Geometry: final body of the model. Coordinates: model frame, mm. A direction names the side the tool comes from. Coordinates: 2 decimals unless noted, no trailing zeros. Loops run counter-clockwise (first coordinate to the right, second up) from the corner with the lowest first, then second, coordinate; pieces in that order, holes last. Notation, with made-up numbers: (57.25, 10.5) - (79.25, 10.5) arc R21 ccw to (79.25, 46.5) - close; hole circle Ø6 at (26, -19). An arc over 180 degrees is marked (long way). Put each result on its own line as item: value. Start each with the question number.
1) Reachability of faces 3 (the cylindrical face through (-25, 16, 2)), 4 (the flat face through (-2, 1, 5)), 5 (the flat face through (-124, -41, 2)), 6 (the flat face through (95, 0, 2)), 7 (the flat face through (-120, -66, 2)) from +Z, -Z, +X, -X, +Y, -Y: full face, straight path, thin tool, end or side. Return the list, or none.
2) Material intervals for line 1 along X through (y, z) = (2.5, 4.7); line 2 along X through (y, z) = (-15, 4.5); line 3 along X through (y, z) = (-39, 0.7), sorted ascending. Write a range as from..to.
3) Section C-C on y = -20.5. Output: boundary loops of the cut face in (x, z), and give its area (3 significant figures).
4) Draft query along Y for faces 1 (the flat face through (120, 65, 2)), 2 (the flat face through (103, -2.2, 2)). Return one class per face: +Y half, -Y half, draft (parallel to the pull), parting line (faces both ways), or undercut.
5) Contact query for flat-ended pins moving along their axis: pin 1 Ø3 at (x, y) = (-37.5, -70.5) entering from +Z; pin 2 Ø5.5 at (x, y) = (-92, 23.5) entering from -Z; pin 3 Ø0.8 at (y, z) = (-3, 1.5) entering from -X; pin 4 Ø2.5 at (y, z) = (-2.5, 3) entering from +X. Output: stop coordinate, or through.
6) Section B-B on x = -12. Output: boundary loops of the cut face in (y, z), and give its area (3 significant figures).
7) Section A-A on y = 12. Output: boundary loops of the cut face in (x, z), and give its area (3 significant figures).
8) Section D-D on x = 91. Output: boundary loops of the cut face in (y, z), and give its area (3 significant figures).
```python
from build123d import *

# Parameters (mm, degrees)
SKETCH1_W           = 240
SKETCH1_H           = 151
BOSS_EXTRUDE1_DEPTH = 5
SKETCH2_R           = 1.25
CUT_EXTRUDE1_DEPTH  = 5
CUT_EXTRUDE2_DEPTH  = 10
SKETCH7_R           = 2
CUT_EXTRUDE4_DEPTH  = 10
SKETCH9_W           = 4
SKETCH9_H           = 30
BOSS_EXTRUDE2_DEPTH = 5
CUT_EXTRUDE6_DEPTH  = 5
SKETCH13_R          = 21
CUT_EXTRUDE9_DEPTH  = 10
SKETCH15_R          = 1.75
CUT_EXTRUDE11_DEPTH = 10
SKETCH16_R          = 1.75
CUT_EXTRUDE12_DEPTH = 10
SKETCH17_R          = 1.75
CUT_EXTRUDE13_DEPTH = 10
SKETCH20_W          = 24.2
SKETCH20_H          = 30.2
CUT_EXTRUDE14_DEPTH = 10
SKETCH21_R          = 5.25
CUT_EXTRUDE15_DEPTH = 5
SKETCH22_R          = 1
CUT_EXTRUDE16_DEPTH = 5
SKETCH23_R          = 5.25
CUT_EXTRUDE17_DEPTH = 10


with BuildPart() as part:
    # Sketch1 → Boss-Extrude1 (new body)
    with BuildSketch(Plane.XY):
        Rectangle(SKETCH1_W, SKETCH1_H)
    extrude(amount=BOSS_EXTRUDE1_DEPTH)

    # Sketch2 → Cut-Extrude1 (cut)
    with BuildSketch(Plane(origin=(0, 0, 0), x_dir=(-1, 0, 0), z_dir=(0, 0, -1))):
        with Locations(Location((-20, 42, 0), (0, 0, 180))):
            Circle(SKETCH2_R)
        with Locations((28, 28)):
            Circle(SKETCH2_R)
        with Locations(Location((20, 42, 0), (0, 0, 180))):
            Circle(SKETCH2_R)
        with Locations((-28, 28)):
            Circle(SKETCH2_R)
        with Locations(Location((-28, -28, 0), (0, 0, 180))):
            Circle(SKETCH2_R)
        with Locations((20, -42)):
            Circle(SKETCH2_R)
        with Locations(Location((28, -28, 0), (0, 0, 180))):
            Circle(SKETCH2_R)
        with Locations((-20, -42)):
            Circle(SKETCH2_R)
    extrude(amount=-CUT_EXTRUDE1_DEPTH, mode=Mode.SUBTRACT)

    # Sketch5 → Cut-Extrude2 (cut)
    with BuildSketch(Plane(origin=(0, 0, 0), x_dir=(-1, 0, 0), z_dir=(0, 0, -1))):
        with BuildLine():
            Line((18.5, -10.5), (18.5, 9.5))
            ThreePointArc((18.5, 9.5), (25, 16), (31.5, 9.5))
            Line((31.5, 9.5), (31.5, -10.5))
            ThreePointArc((31.5, -10.5), (25, -17), (18.5, -10.5))
        make_face()
        with BuildLine():
            Line((-18.5, -10.5), (-18.5, 9.5))
            ThreePointArc((-18.5, 9.5), (-25, 16), (-31.5, 9.5))
            Line((-31.5, 9.5), (-31.5, -10.5))
            ThreePointArc((-31.5, -10.5), (-25, -17), (-18.5, -10.5))
        make_face()
    extrude(amount=-CUT_EXTRUDE2_DEPTH, mode=Mode.SUBTRACT)

    # Sketch7 → Cut-Extrude4 (cut)
    with BuildSketch(Plane(origin=(0, 0, 0), x_dir=(-1, 0, 0), z_dir=(0, 0, -1))):
        with Locations((29.207613065, 40.217347852)):
            Circle(SKETCH7_R)
        with Locations((29.207613065, -40.217347852)):
            Circle(SKETCH7_R)
        with Locations(Location((-29.207613065, -40.217347852, 0), (0, 0, 180))):
            Circle(SKETCH7_R)
        with Locations(Location((-29.207613065, 40.217347852, 0), (0, 0, 180))):
            Circle(SKETCH7_R)
    extrude(amount=-CUT_EXTRUDE4_DEPTH, mode=Mode.SUBTRACT)

    # Sketch9 → Boss-Extrude2 (add)
    with BuildSketch(Plane(origin=(0, 0, 0), x_dir=(-1, 0, 0), z_dir=(0, 0, -1))):
        with Locations((122, 40.5)):
            Rectangle(SKETCH9_W, SKETCH9_H)
        with Locations((122, -40.5)):
            Rectangle(SKETCH9_W, SKETCH9_H)
        with Locations((-122, -40.5)):
            Rectangle(SKETCH9_W, SKETCH9_H)
        with Locations((-122, 40.5)):
            Rectangle(SKETCH9_W, SKETCH9_H)
    extrude(amount=-BOSS_EXTRUDE2_DEPTH)

    # Sketch10 → Cut-Extrude6 (cut)
    with BuildSketch(Plane(origin=(0, 0, 0), x_dir=(-1, 0, 0), z_dir=(0, 0, -1))):
        Polygon((-120, 2.2), (-115, 2.2), (-115, 3.7), (-111.7, 3.7), (-111.7, 2.2), (-95, 2.2), (-95, -2.2), (-111.7, -2.2), (-111.7, -3.7), (-115, -3.7), (-115, -2.2), (-120, -2.2), align=None)
        Polygon((115, -2.2), (120, -2.2), (120, 2.2), (115, 2.2), (115, 3.7), (111.7, 3.7), (111.7, 2.2), (95, 2.2), (95, -2.2), (111.7, -2.2), (111.7, -3.7), (115, -3.7), align=None)
    extrude(amount=-CUT_EXTRUDE6_DEPTH, mode=Mode.SUBTRACT)

    # Sketch13 → Cut-Extrude9 (cut)
    with BuildSketch(Plane(origin=(0, 0, 0), x_dir=(-1, 0, 0), z_dir=(0, 0, -1))):
        with Locations((-85, 35.5)):
            Circle(SKETCH13_R)
    extrude(amount=-CUT_EXTRUDE9_DEPTH, mode=Mode.SUBTRACT)

    # Sketch15 → Cut-Extrude11 (cut)
    with BuildSketch(Plane(origin=(0, 0, 0), x_dir=(-1, 0, 0), z_dir=(0, 0, -1))):
        with Locations((-34, -40.5)):
            Circle(SKETCH15_R)
    extrude(amount=-CUT_EXTRUDE11_DEPTH, mode=Mode.SUBTRACT)

    # Sketch16 → Cut-Extrude12 (cut)
    with BuildSketch(Plane(origin=(0, 0, 0), x_dir=(-1, 0, 0), z_dir=(0, 0, -1))):
        with Locations((-42, 25.5)):
            Circle(SKETCH16_R)
        with Locations((87, -70.5)):
            Circle(SKETCH16_R)
        with Locations((27.5, -70.5)):
            Circle(SKETCH16_R)
        with Locations((87, 18.5)):
            Circle(SKETCH16_R)
        with Locations((27.5, 18.5)):
            Circle(SKETCH16_R)
        with Locations((-42, 30.5)):
            Circle(SKETCH16_R)
        with Locations((27.5, 23.5)):
            Circle(SKETCH16_R)
        with Locations((87, -65.5)):
            Circle(SKETCH16_R)
        with Locations((87, 23.5)):
            Circle(SKETCH16_R)
        with Locations((27.5, -65.5)):
            Circle(SKETCH16_R)
        with Locations((87, -60.5)):
            Circle(SKETCH16_R)
        with Locations((87, 28.5)):
            Circle(SKETCH16_R)
        with Locations((27.5, -60.5)):
            Circle(SKETCH16_R)
        with Locations((32.5, -70.5)):
            Circle(SKETCH16_R)
        with Locations((92, -70.5)):
            Circle(SKETCH16_R)
        with Locations((32.5, -65.5)):
            Circle(SKETCH16_R)
        with Locations((32.5, -60.5)):
            Circle(SKETCH16_R)
        with Locations((92, -65.5)):
            Circle(SKETCH16_R)
        with Locations((92, -60.5)):
            Circle(SKETCH16_R)
        with Locations((32.5, 18.5)):
            Circle(SKETCH16_R)
        with Locations((32.5, 23.5)):
            Circle(SKETCH16_R)
        with Locations((92, 23.5)):
            Circle(SKETCH16_R)
        with Locations((92, 18.5)):
            Circle(SKETCH16_R)
        with Locations((92, 28.5)):
            Circle(SKETCH16_R)
        with Locations((37.5, -70.5)):
            Circle(SKETCH16_R)
        with Locations((97, -70.5)):
            Circle(SKETCH16_R)
        with Locations((37.5, -65.5)):
            Circle(SKETCH16_R)
        with Locations((37.5, -60.5)):
            Circle(SKETCH16_R)
        with Locations((97, -65.5)):
            Circle(SKETCH16_R)
        with Locations((97, -60.5)):
            Circle(SKETCH16_R)
        with Locations((37.5, 18.5)):
            Circle(SKETCH16_R)
        with Locations((37.5, 23.5)):
            Circle(SKETCH16_R)
        with Locations((97, 23.5)):
            Circle(SKETCH16_R)
        with Locations((97, 18.5)):
            Circle(SKETCH16_R)
        with Locations((97, 28.5)):
            Circle(SKETCH16_R)
    extrude(amount=-CUT_EXTRUDE12_DEPTH, mode=Mode.SUBTRACT)

    # Sketch17 → Cut-Extrude13 (cut)
    with BuildSketch(Plane(origin=(0, 0, 0), x_dir=(-1, 0, 0), z_dir=(0, 0, -1))):
        with Locations((-116, -70.5)):
            Circle(SKETCH17_R)
        with Locations((-116, -50.5)):
            Circle(SKETCH17_R)
        with Locations((-1, -50.5)):
            Circle(SKETCH17_R)
        with Locations((-1, -70.5)):
            Circle(SKETCH17_R)
        with Locations((-116, -45.5)):
            Circle(SKETCH17_R)
        with Locations((-116, -65.5)):
            Circle(SKETCH17_R)
        with Locations((-1, -45.5)):
            Circle(SKETCH17_R)
        with Locations((-1, -65.5)):
            Circle(SKETCH17_R)
        with Locations((-116, -40.5)):
            Circle(SKETCH17_R)
        with Locations((-116, -60.5)):
            Circle(SKETCH17_R)
        with Locations((-1, -40.5)):
            Circle(SKETCH17_R)
        with Locations((-1, -60.5)):
            Circle(SKETCH17_R)
    extrude(amount=-CUT_EXTRUDE13_DEPTH, mode=Mode.SUBTRACT)

    # Sketch20 → Cut-Extrude14 (cut)
    with BuildSketch(Plane(origin=(0, 0, 0), x_dir=(-1, 0, 0), z_dir=(0, 0, -1))):
        with Locations((102.9, 55.4)):
            Rectangle(SKETCH20_W, SKETCH20_H)
    extrude(amount=-CUT_EXTRUDE14_DEPTH, mode=Mode.SUBTRACT)

    # Sketch21 → Cut-Extrude15 (cut)
    with BuildSketch(Plane(origin=(0, 0, 0), x_dir=(-1, 0, 0), z_dir=(0, 0, -1))):
        with Locations((13.963511127, -61)):
            Circle(SKETCH21_R)
    extrude(amount=-CUT_EXTRUDE15_DEPTH, mode=Mode.SUBTRACT)

    # Sketch22 → Cut-Extrude16 (cut)
    with BuildSketch(Plane(origin=(0, 0, 0), x_dir=(-1, 0, 0), z_dir=(0, 0, -1))):
        with Locations((23.463511127, -53)):
            Circle(SKETCH22_R)
        with Locations((23.463511127, -69)):
            Circle(SKETCH22_R)
        with Locations((4.463511127, -53)):
            Circle(SKETCH22_R)
        with Locations((4.463511127, -69)):
            Circle(SKETCH22_R)
    extrude(amount=-CUT_EXTRUDE16_DEPTH, mode=Mode.SUBTRACT)

    # Sketch23 → Cut-Extrude17 (cut)
    with BuildSketch(Plane(origin=(0, 0, 0), x_dir=(-1, 0, 0), z_dir=(0, 0, -1))):
        with Locations((0, 61.653760848)):
            Circle(SKETCH23_R)
    extrude(amount=-CUT_EXTRUDE17_DEPTH, mode=Mode.SUBTRACT)


solid = part.part
```
Answer block:
1. face 3: +Z, -Z
1. face 4: +Z, +X, -X, +Y, -Y
1. face 5: +Z, -Z, -X, +Y, -Y
1. face 6: +Z, -Z, +X
1. face 7: +Z, -Z, -X, -Y
2. line 1: x = -120..-115, -111.7..-31.5, -18.5..18.5, 31.5..111.7, 115..120
2. line 2: x = -120..-29.69, -20.31..20.31, 29.69..120
2. line 3: x = -124..-30.79, -27.62..0.1, 1.9..27.62, 30.79..33.1, 34.9..115.1, 116.9..124
3. outline: (-120, 0) - (120, 0) - (120, 5) - (-120, 5) - close
3. area: 1,200 mm²
4. face 1: draft
4. face 2: undercut
5. pin 1: passes through
5. pin 2: stops at z = 0
5. pin 3: stops at x = -120
5. pin 4: stops at x = 120
6. outline: (-75.5, 0) - (-65.87, 0) - (-65.87, 5) - (-75.5, 5) - close; (-56.13, 0) - (75.5, 0) - (75.5, 5) - (-56.13, 5) - close
6. area: 706 mm²
7. outline: (-120, 0) - (-31, 0) - (-31, 5) - (-120, 5) - close; (-19, 0) - (19, 0) - (19, 5) - (-19, 5) - close; (31, 0) - (120, 0) - (120, 5) - (31, 5) - close
7. area: 1,080 mm²
8. outline: (-75.5, 0) - (15.38, 0) - (15.38, 5) - (-75.5, 5) - close; (55.62, 0) - (75.5, 0) - (75.5, 5) - (55.62, 5) - close
8. area: 554 mm²
